Design review of the part shown in the three views and the two pictorial views. Dimensions are in mm from the part's minimum x, y and z. Coordinates: 2 decimals unless noted, no trailing zeros. Loops run counter-clockwise (first coordinate to the right, second up) from the corner with the lowest first, then second, coordinate; pieces in that order, holes last.
Q1. Wall thickness on probe 1 along Y at (x, z) = (38, 0.75); probe 2 along X at (y, z) = (33, 0.95); probe 3 along Y at (x, z) = (44.5, 0.4): over which ranges is each line inside the solid? List them lowest first.
Q2. Add section D-D on z = 0.2. Give the boundary of the cut face in (x, y), and give its area (3 significant figures).
Q3. Add section A-A on x = 38. Give the boundary of the cut face in (y, z), and give its area (3 significant figures).
Q4. Add section B-B on y = 18. Give the boundary of the cut face in (x, z).
Q5. Add section C-C on x = 17. Give the boundary of the cut face in (y, z).
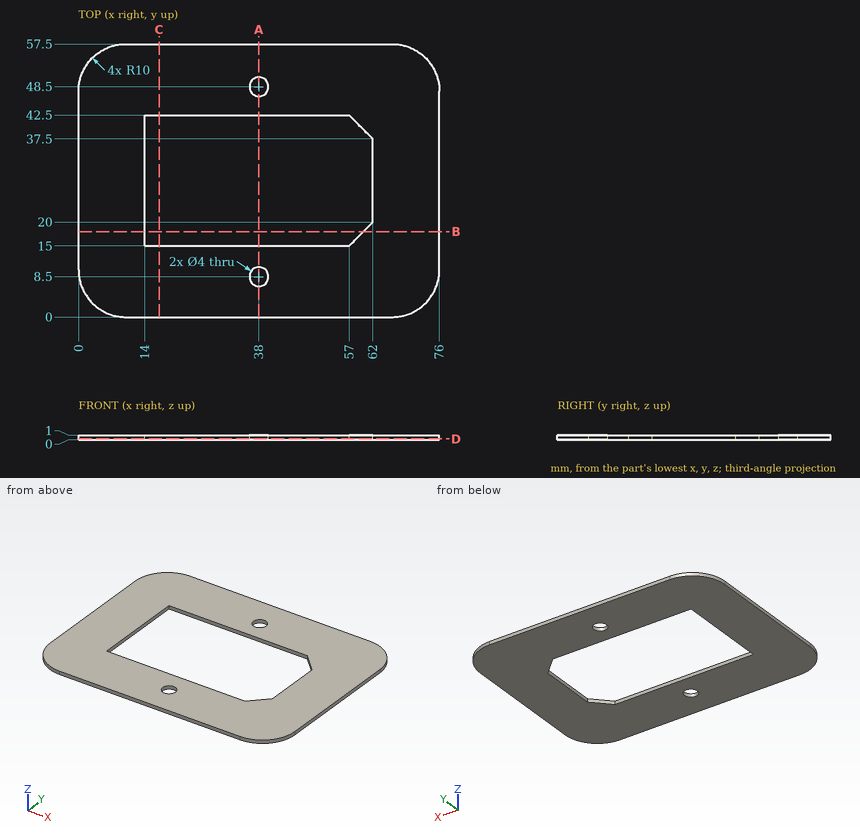
Entries:
1. probe 1: y = 0 to 6.5, 10.5 to 15, 42.5 to 46.5, 50.5 to 57.5
1. probe 2: x = 0 to 14, 62 to 76
1. probe 3: y = 0 to 15, 42.5 to 57.5
2. outline: (0, 10) arc R10 ccw to (10, 0) - (66, 0) arc R10 ccw to (76, 10) - (76, 47.5) arc R10 ccw to (66, 57.5) - (10, 57.5) arc R10 ccw to (0, 47.5) - close; hole (14, 15) - (57, 15) - (62, 20) - (62, 37.5) - (57, 42.5) - (14, 42.5) - close; hole circle Ø4 at (38, 8.5); hole circle Ø4 at (38, 48.5)
2. area: 2,960 mm2
3. outline: (0, 0) - (6.5, 0) - (6.5, 1) - (0, 1) - close; (10.5, 0) - (15, 0) - (15, 1) - (10.5, 1) - close; (42.5, 0) - (46.5, 0) - (46.5, 1) - (42.5, 1) - close; (50.5, 0) - (57.5, 0) - (57.5, 1) - (50.5, 1) - close
3. area: 22.0 mm2
4. outline: (0, 0) - (14, 0) - (14, 1) - (0, 1) - close; (60, 0) - (76, 0) - (76, 1) - (60, 1) - close
5. outline: (0, 0) - (15, 0) - (15, 1) - (0, 1) - close; (42.5, 0) - (57.5, 0) - (57.5, 1) - (42.5, 1) - close
